Can you work these out from the model? Positions are in its coordinate system, mm. Face numbers are marked on the shaded views. A direction names the side the tool comes from. Coordinates: 2 decimals unless noted, no trailing zeros. Write each loop counter-clockwise with the first axis right and the second up, starting at its lowest first coordinate (ties: lowest second). Pieces come first, ordered by that corner, then holes. Notation, with made-up numbers: M 78.25,43.5 L 102.25,43.5 A29 ccw 102.25,70.5 Z; hole C 81.5,-8.75 d3. An arc over 180 degrees is marked long. Use one line per item in the form item = value. Start each with the question number.
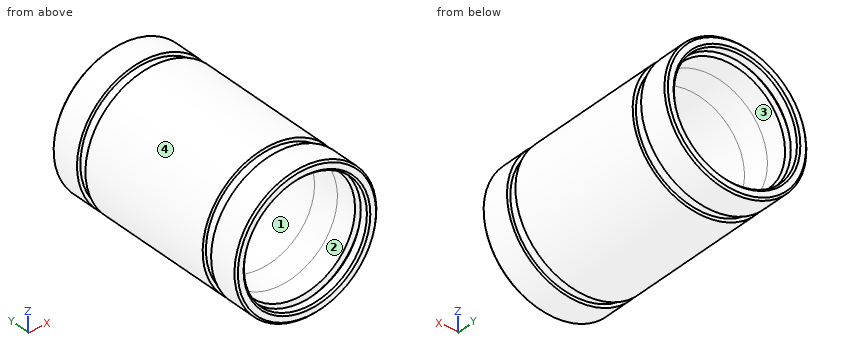
```python
from build123d import *


with BuildPart() as part:
    # Sketch1 → Revolve1 (revolve)
    with BuildSketch(Plane(origin=(0, 0, 0), x_dir=(0, 0, -1), z_dir=(1, 0, 0))):
        Polygon((6.7, 12), (7.3, 12), (7.5, 11.8), (7.5, 8.75), (7.15, 8.75), (7.15, 7.65), (7.5, 7.65), (7.5, -7.65), (7.15, -7.65), (7.15, -8.75), (7.5, -8.75), (7.5, -11.8), (7.3, -12), (6.7, -12), (6.5, -11.8), (6.5, -11), (7, -11), (7, -10.5), (6.3, -10.5), (6.3, -8.2), (5.9, -5.7), (5.9, 5.7), (6.3, 8.2), (6.3, 10.5), (7, 10.5), (7, 11), (6.5, 11), (6.5, 11.8), align=None)
    revolve(axis=Axis((0, 12, 0), (0, -1, 0)))


solid = part.part
```
1) Suppose I cut it at A-A on y = -2.75. Please give me the cut outline in (x, z), and give its area (3 significant figures).
2) If we mould it in two halves opening along Z, with no side actions, what happens to the marked faces 3 and 4? For each: +Z half, -Z half, draft (parallel to the pull), parting line (faces both ways), or undercut.
3) Please list where these lines run through material, in increasing order: line 1 (X direction, y = -3, z = 0); line 2 (Z direction, x = 0.25, y = 9.25); line 3 (Z direction, x = -0.25, y = 5.25).
4) Will these pins go through, and if not, where does the flat tip stop? pin 1 Ø1.5 at (y, z) = (4, -4) entering from -X; pin 2 Ø2 at (x, y) = (-2.5, 0.5) entering from -Z; pin 3 Ø5 at (y, z) = (-6.5, 3.5) entering from -X.
5) Which directions (+Z, -Z, +X, -X, +Y, -Y) give clear straight access to the entire face, cutting with the end or side of a thin tool? Please do the marked faces 1 and 2.
Computed values:
q1.outline = C 0,0 d15; hole C 0,0 d11.8
q1.area = 67.4 mm²
q2.face_3 = undercut
q2.face_4 = parting line
q3.line_1 = -7.5 to -5.9, 5.9 to 7.5
q3.line_2 = -7.5 to -6.3, 6.3 to 7.5
q3.line_3 = -7.5 to -5.89, 5.89 to 7.5
q4.pin_1 = -6.76
q4.pin_2 = -7.35
q4.pin_3 = -7.43
q5.face_1 = +Y, -Y
q5.face_2 = -Y
